```python
from build123d import *

# Parameters (mm, degrees)
SKETCH1_R           = 1.75
SKETCH1_R_2         = 8.5
SKETCH1_R_3         = 1.5
BOSS_EXTRUDE1_DEPTH = 2.7
FILLET1_R           = 3


with BuildPart() as part:
    # Sketch1 → Boss-Extrude1 (new body)
    with BuildSketch(Plane.XY):
        with BuildLine():
            Line((10.487675588, 31), (-10.487675588, 31))
            Line((-10.487675588, 31), (-20.108076211, 14.336977332))
            ThreePointArc((-20.108076211, 14.336977332), (-20.407777479, 13.613434467), (-20.51, 12.836977332))
            Line((-20.51, 12.836977332), (-20.51, -12.596152423))
            ThreePointArc((-20.51, -12.596152423), (-20.407777479, -13.372609558), (-20.108076211, -14.096152423))
            Line((-20.108076211, -14.096152423), (-10.348635262, -31))
            Line((-10.348635262, -31), (10.348635262, -31))
            Line((10.348635262, -31), (20.108076211, -14.096152423))
            ThreePointArc((20.108076211, -14.096152423), (20.407777479, -13.372609558), (20.51, -12.596152423))
            Line((20.51, -12.596152423), (20.51, 12.836977332))
            ThreePointArc((20.51, 12.836977332), (20.407777479, 13.613434467), (20.108076211, 14.336977332))
            Line((20.108076211, 14.336977332), (10.487675588, 31))
        make_face()
        with Locations(Location((-6, -27, 0), (0, 0, 180))):
            Circle(SKETCH1_R, mode=Mode.SUBTRACT)
        with Locations(Location((6, -27, 0), (0, 0, 180))):
            Circle(SKETCH1_R, mode=Mode.SUBTRACT)
        with Locations(Location((7.5, -13.4, 0), (0, 0, 180))):
            Circle(SKETCH1_R_2, mode=Mode.SUBTRACT)
        with BuildLine():
            ThreePointArc((-4.5, -13.4), (-8.54, -17.44), (-12.58, -13.4))
            Line((-12.58, -13.4), (-12.58, 1.685368783))
            ThreePointArc((-12.58, 1.685368783), (-10.18215631, 2.859423407), (-8.730303993, 5.1))
            Line((-8.730303993, 5.1), (8.729875369, 5.1))
            ThreePointArc((8.729875369, 5.1), (10.179804764, 2.860963681), (12.574584064, 1.685969643))
            ThreePointArc((12.574584064, 1.685969643), (14.121431526, -0.726790857), (11.622623122, -2.13039581))
            ThreePointArc((11.622623122, -2.13039581), (11.545720037, -2.104624526), (11.469942926, -2.075709596))
            ThreePointArc((11.469942926, -2.075709596), (0.558793877, -3.611248417), (-4.5, -13.4))
        make_face(mode=Mode.SUBTRACT)
        with Locations(Location((-13.5, 6.6, 0), (0, 0, 180))):
            Circle(SKETCH1_R_3, mode=Mode.SUBTRACT)
        with BuildLine():
            Line((8.729875369, 8.1), (-8.730303993, 8.1))
            ThreePointArc((-8.730303993, 8.1), (-10.179901517, 10.338575405), (-12.574074074, 11.513518208))
            ThreePointArc((-12.574074074, 11.513518208), (-0.00020804, 20.099999998), (12.57392263, 11.513905748))
            ThreePointArc((12.57392263, 11.513905748), (10.179553129, 10.338812856), (8.729875369, 8.1))
        make_face(mode=Mode.SUBTRACT)
        with Locations(Location((-5.24, 27, 0), (0, 0, 180))):
            Circle(SKETCH1_R_3, mode=Mode.SUBTRACT)
        with Locations(Location((13.5, 6.6, 0), (0, 0, 180))):
            Circle(SKETCH1_R_3, mode=Mode.SUBTRACT)
        with Locations(Location((5.24, 27, 0), (0, 0, 180))):
            Circle(SKETCH1_R_3, mode=Mode.SUBTRACT)
    extrude(amount=BOSS_EXTRUDE1_DEPTH)

    # Fillet1
    fillet1_edges = [part.edges().sort_by_distance(p)[0] for p in [
        (-10.487675588, 31, 1.35),
        (10.487675588, 31, 1.35),
        (10.348635262, -31, 1.35),
        (-10.348635262, -31, 1.35),
    ]]
    fillet(fillet1_edges, radius=FILLET1_R)


solid = part.part
```
Geometry check sheet. Reference: the model listing, model coordinates, mm. A direction names the side the tool comes from. Give positions to 0.01 mm unless a question says otherwise; leave off trailing zeros. Write each loop counter-clockwise with the first axis right and the second up, starting at its lowest first coordinate (ties: lowest second). Pieces come first, ordered by that corner, then holes.
1) Material ranges on L1, parallel to X at y = 6.6, z = 2; L2, parallel to Y at x = -6, z = 1.5; L3, parallel to X at y = -16, z = 1.4, recorded low to high.
2) Section check B-B, the plane x = 3. Record the boundary of the cut face in (y, z).
3) Release check for a two-part mould opening along X. For faces 1 (the cylindrical face through (10.237, 30.609, 1.369)), 2 (the flat face through (-15.724, -21.69, 1.331)), 3 (the flat face through (-12.58, -6, 1)) record: pulls with the +X half, pulls with the -X half, needs draft (parallel to the pull), parting line crosses it, or undercut.
4) Section check D-D, the plane x = -5.5. Record the boundary of the cut face in (y, z).
5) Section check A-A, the plane y = 6.6. Record the boundary of the cut face in (x, z).
6) Access from +Z, -Z, +X, -X, +Y, -Y to the whole of each face (thin tool, end or side, straight path). Record for faces 4 (the flat face through (-15.67, 22.02, 1.33)), 5 (the cylindrical face through (10.15, 2.89, 1.33)).
7) Section check C-C, the plane y = 13.5. Record the boundary of the cut face in (x, z).
Computed:
1. L1: x = -20.51 to -15, -12 to 12, 15 to 20.51
1. L2: y = -31 to -28.75, -25.25 to -16.54, 5.1 to 8.1, 18.69 to 25.71, 28.29 to 31
1. L3: x = -19.01 to -11.63, -5.45 to -0.59, 15.59 to 19.01
2. outline: (-31, 0) - (-20.61, 0) - (-20.61, 2.7) - (-31, 2.7) - close; (-6.19, 0) - (-2.28, 0) - (-2.28, 2.7) - (-6.19, 2.7) - close; (5.1, 0) - (8.1, 0) - (8.1, 2.7) - (5.1, 2.7) - close; (19.76, 0) - (31, 0) - (31, 2.7) - (19.76, 2.7) - close
3. face 1: pulls with the +X half
3. face 2: pulls with the -X half
3. face 3: undercut
4. outline: (-31, 0) - (-28.68, 0) - (-28.68, 2.7) - (-31, 2.7) - close; (-25.32, 0) - (-16.06, 0) - (-16.06, 2.7) - (-25.32, 2.7) - close; (5.1, 0) - (8.1, 0) - (8.1, 2.7) - (5.1, 2.7) - close; (18.93, 0) - (25.52, 0) - (25.52, 2.7) - (18.93, 2.7) - close; (28.48, 0) - (31, 0) - (31, 2.7) - (28.48, 2.7) - close
5. outline: (-20.51, 0) - (-15, 0) - (-15, 2.7) - (-20.51, 2.7) - close; (-12, 0) - (12, 0) - (12, 2.7) - (-12, 2.7) - close; (15, 0) - (20.51, 0) - (20.51, 2.7) - (15, 2.7) - close
6. face 4: +Z, -Z, -X, +Y
6. face 5: +Z, -Z
7. outline: (-20.44, 0) - (-11.6, 0) - (-11.6, 2.7) - (-20.44, 2.7) - close; (11.6, 0) - (20.44, 0) - (20.44, 2.7) - (11.6, 2.7) - close
